Can you work these out from the model? Positions are in its coordinate system, mm. A direction names the side the tool comes from. Coordinates: 2 decimals unless noted, no trailing zeros. Write each loop counter-clockwise with the first axis right and the second up, starting at its lowest first coordinate (ties: lowest second). Pieces come first, ordered by that corner, then holes. Notation, with made-up numbers: (62.25, -7) - (85.25, -7) arc R22 ccw to (85.25, 24) - close; hole circle Ø2 at (37.25, 71). An arc over 180 degrees is marked (long way). Use one line per item in the form item = value. Start each with the question number.
(1) If we section it at C-C on y = 0: Please give me the cut outline in (x, z).
(2) If I drill on probe 1 along X at (y, z) = (-6, 30); probe 2 along Y at (x, z) = (10, 18); probe 3 along Y at (x, z) = (-13, 19), over which ranges is the centre line in solid material (lowest first)? Write a range as from..to.
(3) If we section it at B-B on x = 0: Please give me the cut outline in (y, z), then the cut area to 3 significant figures.
(4) If we section it at D-D on z = 3: Please give me the cut outline in (x, y), then the cut area to 3 significant figures.
(5) If we section it at A-A on z = 30: Please give me the cut outline in (x, y), then the cut area to 3 significant figures.
(6) Thinking about a two-plate mould opening in X: for faces 5 (the face through (23.846, 7.509, 7.605)), 6 (the face through (0, 0, 25)), 7 (the face through (-11, -11, 10)), 8 (the face through (15, 15, 10)), which applies, pulls with the +X half, pulls with the -X half, needs draft (parallel to the pull), parting line crosses it, or undercut?
(7) For pin 1 Ø7 at (x, z) = (-5.5, 27.5) entering from +Y; pin 2 Ø4.5 at (x, z) = (-6.5, 29.5) entering from -Y; pin 3 Ø3 at (x, z) = (10, 21) entering from -Y, each with a flat end and sliding along its axis, tell me the tip position at first contact or that it passes through.
(8) On a 3-axis mill with a long thin cutter (end or side, diameter ignored), from which of +Z, -Z, +X, -X, +Y, -Y can I reach the whole of each face in a straight line? I mean faces 1 (the face through (0, 3.1, 29)), 2 (the face through (-5.961, -26.846, 18.803)), 3 (the face through (-20, -6, 30)), 4 (the face through (12.1, -22.3, 15)). Say none if no direction works.
Solid Edge part; units mm, degrees
sketch "Sketch1" plane through (0, 0, 0) normal (0, -1, 0) x (1, 0, 0)
  line L0 (0, 0) -> (25, 0)
  line L1 (25, 0) -> (25, 15)
  line L2 (25, 15) -> (27.5, 15)
  line L3 (27.5, 15) -> (27.5, 25)
  line L4 (27.5, 25) -> (0, 25)
  dimension "D1" = 25
revolve "RevolvedProtrusion1" add sketch "Sketch1" angle 360 about axis through (0, 0, 0) along (0, 0, 1)
chamfer "Chamfer1" distance 2.5 angle 45 1 edges at (-27.5, 0, 25)
sketch "Sketch2" plane through (0, 0, 25) normal (0, 0, 1) x (1, 0, 0)
  line L0 (-20, 3.1) -> (20, 3.1)
  line L1 (20, 3.1) -> (20, 9.1)
  line L2 (20, 9.1) -> (-20, 9.1)
  line L3 (-20, 9.1) -> (-20, 3.1)
  line L4 (-20, -9.1) -> (20, -9.1)
  line L5 (20, -9.1) -> (20, -3.1)
  line L6 (20, -3.1) -> (-20, -3.1)
  line L7 (-20, -3.1) -> (-20, -9.1)
  dimension "D1" = 20
  dimension "D2" = 20
extrude "ExtrudedProtrusion_1" add sketch "Sketch2" along normal blind 10
hole "Hole_1" at (-10, -9.1, 30) direction (0, 1, 0) diameter 6 end through all
hole "Hole1" at (10, -9.1, 30) direction (0, 1, 0) diameter 6 end through all
chamfer "Chamfer_2" distance 1 angle 45 4 edges at (0, -3.1, 35) (0, -9.1, 35) (0, 3.1, 35) (0, 9.1, 35)
hole "Hole_3" at (-13, -13, 25) direction (0, 0, -1) diameter 5 end up to next counterbore diameter 8 counterbore depth 15
hole "Hole2" at (-13, 13, 25) direction (0, 0, -1) diameter 5 end up to next counterbore diameter 8 counterbore depth 15
hole "Hole3" at (13, -13, 25) direction (0, 0, -1) diameter 5 end up to next counterbore diameter 8 counterbore depth 15
hole "Hole4" at (13, 13, 25) direction (0, 0, -1) diameter 5 end up to next counterbore diameter 8 counterbore depth 15
properties material "Polyethylene, low density"
Reported:
q1.outline = (-27.5, 15) - (-25, 15) - (-25, 0) - (25, 0) - (25, 15) - (27.5, 15) - (27.5, 22.5) - (25, 25) - (-25, 25) - (-27.5, 22.5) - close
q2.probe_1 = -20..-13, -7..7, 13..20
q2.probe_2 = -25.62..-15.65, -10.35..10.35, 15.65..25.62
q2.probe_3 = -24.23..-17, -9..9, 17..24.23
q3.outline = (-27.5, 15) - (-25, 15) - (-25, 0) - (25, 0) - (25, 15) - (27.5, 15) - (27.5, 22.5) - (25, 25) - (9.1, 25) - (9.1, 34) - (8.1, 35) - (4.1, 35) - (3.1, 34) - (3.1, 25) - (-3.1, 25) - (-3.1, 34) - (-4.1, 35) - (-8.1, 35) - (-9.1, 34) - (-9.1, 25) - (-25, 25) - (-27.5, 22.5) - close
q3.area = 1,410 mm2
q4.outline = circle Ø50 at (0, 0); hole circle Ø5 at (-13, -13); hole circle Ø5 at (-13, 13); hole circle Ø5 at (13, -13); hole circle Ø5 at (13, 13)
q4.area = 1,880 mm2
q5.outline = (-20, -9.1) - (-13, -9.1) - (-13, -3.1) - (-20, -3.1) - close; (-20, 3.1) - (-13, 3.1) - (-13, 9.1) - (-20, 9.1) - close; (-7, -9.1) - (7, -9.1) - (7, -3.1) - (-7, -3.1) - close; (-7, 3.1) - (7, 3.1) - (7, 9.1) - (-7, 9.1) - close; (13, -9.1) - (20, -9.1) - (20, -3.1) - (13, -3.1) - close; (13, 3.1) - (20, 3.1) - (20, 9.1) - (13, 9.1) - close
q5.area = 336 mm2
q6.face_5 = parting line crosses it
q6.face_6 = needs draft
q6.face_7 = undercut
q6.face_8 = undercut
q7.pin_1 = 25.48
q7.pin_2 = -9.1
q7.pin_3 = -26.15
q8.face_1 = +Z, +X, -X
q8.face_2 = +Z, -Z
q8.face_3 = +Z, -X, +Y, -Y
q8.face_4 = -Z
